Verification items for the finished model (mm, model axes). Face numbers are marked on the shaded views. A direction names the side the tool comes from. Round coordinates to 2 decimals unless told otherwise and drop trailing zeros. Order: outer loops, then holes, each group sorted by start corner. A loop starts at its lowest first (then second) coordinate and runs counter-clockwise, first axis right, second up. Notation, with made-up numbers: M 44,65 L 89,65 A23 cw 89,75 Z; hole C -25.75,69 d11. An arc over 180 degrees is marked long. Use one line per item in the form item = value. Start each with the question number.
Item 1: Thickness scan on probe 1 along X at (y, z) = (-225, 49.5); probe 2 along Y at (x, z) = (25.5, 59); probe 3 along Z at (x, y) = (41, -56.5). Record the ranges inside material, lowest first. Write a range as [from, to].
Item 2: Go/stop test with flat-tipped pins: pin 1 Ø15 at (x, z) = (17, 46) entering from -Y; pin 2 Ø6 at (x, y) = (-54.5, -233) entering from -Z; pin 3 Ø25 at (x, z) = (28, 57.5) entering from +Y. Record where each tip stops, or that it passes through.
Item 3: Release check for a two-part mould opening along Y. For the marked faces 1, 2 and 3 record: +Y half, -Y half, draft (parallel to the pull), parting line (faces both ways), or undercut.
Item 4: Cross-section at D-D on y = -314. Enter the section's corners in (x, z), then the cut area to 3 significant figures.
Item 5: Tool access check on the marked faces 4, 5 and 6. Record the directions out of +Z, -Z, +X, -X, +Y, -Y that give a thin tool (end or side, any length) a straight path to the whole face; none if there is none.
Item 6: Cross-section at B-B on x = -210. Enter the section's corners in (y, z).
Item 7: Cross-section at C-C on y = -175. Enter the section's corners in (x, z).
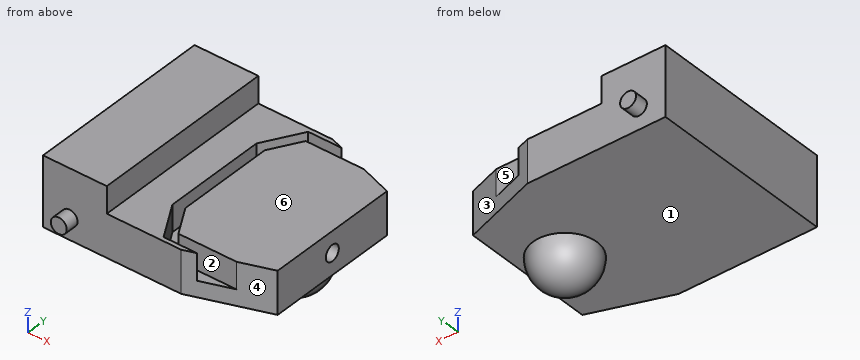
from build123d import *

# Parameters (mm, degrees)
BOSS_EXTRUDE1_DEPTH = 80
SKETCH2_R           = 15
BOSS_EXTRUDE2_DEPTH = 25
BOSS_EXTRUDE3_START = -375
SKETCH2_2_R         = 15
BOSS_EXTRUDE3_DEPTH = 25
SKETCH4_R           = 15
CUT_EXTRUDE1_DEPTH  = 30
CUT_EXTRUDE3_DEPTH  = 50
REVOLVE1_ANGLE      = 180
SKETCH6_W           = 120
SKETCH6_H           = 350
BOSS_EXTRUDE4_DEPTH = 50


with BuildPart() as part:
    # Sketch1 → Boss-Extrude1 (new body)
    with BuildSketch(Plane.XY):
        Polygon((0, 0), (-260, 0), (-260, -350), (0, -350), (141.863078537, -301.267393379), (141.863078537, -48.732606621), align=None)
    extrude(amount=BOSS_EXTRUDE1_DEPTH)

    # Sketch2 → Boss-Extrude2 (add)
    with BuildSketch(Plane.XZ.offset(350)):
        with Locations(Location((-210, 40, 0), (0, 0, 90))):
            Circle(SKETCH2_R)
    extrude(amount=BOSS_EXTRUDE2_DEPTH)

    # Sketch2<2> → Boss-Extrude3 (add)
    with BuildSketch(Plane.XZ.offset(350).offset(BOSS_EXTRUDE3_START)):
        with Locations(Location((-210, 40, 0), (0, 0, 90))):
            Circle(SKETCH2_2_R)
    extrude(amount=BOSS_EXTRUDE3_DEPTH)

    # Sketch4 → Cut-Extrude1 (cut)
    with BuildSketch(Plane(origin=(141.863078537, 0, 0), x_dir=(0, 0, -1), z_dir=(1, 0, 0))):
        with Locations((-40, -175)):
            Circle(SKETCH4_R)
    extrude(amount=-CUT_EXTRUDE1_DEPTH, mode=Mode.SUBTRACT)

    # Sketch5 → Cut-Extrude3 (cut)
    with BuildSketch(Plane.XY.offset(80)):
        Polygon((23.288403945, -342), (-39.585481157, -342), (-80, -272), (-80, -78), (-39.585481157, -8), (23.288403945, -8), (81.509413808, -28), (-28.038475773, -28), (-60, -83.358983849), (-60, -266.641016151), (-28.038475773, -322), (81.509413808, -322), align=None)
    extrude(amount=-CUT_EXTRUDE3_DEPTH, mode=Mode.SUBTRACT)

    # Sketch3 → Revolve1 (revolve)
    with BuildSketch(Plane(origin=(0, 0, 0), x_dir=(-1, 0, 0), z_dir=(0, 0, -1))):
        with BuildLine():
            Line((-11.863078537, -175), (-131.863078537, -175))
            ThreePointArc((-131.863078537, -175), (-71.863078537, -115), (-11.863078537, -175))
        make_face()
    revolve(axis=Axis((141.863078537, -175, 0), (-1, 0, 0)), revolution_arc=REVOLVE1_ANGLE)

    # Sketch6 → Boss-Extrude4 (add)
    with BuildSketch(Plane.XY.offset(80)):
        with Locations((-200, -175)):
            Rectangle(SKETCH6_W, SKETCH6_H)
    extrude(amount=BOSS_EXTRUDE4_DEPTH)


solid = part.part
Output values:
q1.probe_1 = [-260, -80], [-60, 141.86]
q1.probe_2 = [-322, -28]
q1.probe_3 = [0, 80]
q2.pin_1 = -346.74
q2.pin_2 = 0
q2.pin_3 = -5.32
q3.face_1 = draft
q3.face_2 = undercut
q3.face_3 = +Y half
q4.outline = M -260,0 L 104.8,0 L 104.8,80 L -32.66,80 L -32.66,30 L -55.75,30 L -55.75,80 L -140,80 L -140,130 L -260,130 Z
q4.area = 34,000 mm2
q5.face_4 = +Z, -Z, +X, -Y
q5.face_5 = +Z, +X
q5.face_6 = +Z, +X, +Y, -Y
q6.outline = M -375,25 L -350,25 L -350,0 L 0,0 L 0,25 L 25,25 L 25,55 L 0,55 L 0,130 L -350,130 L -350,55 L -375,55 Z
q7.outline = M -260,0 L 11.86,0 A60 ccw 131.86,0 L 141.86,0 L 141.86,25 L 111.86,25 L 111.86,55 L 141.86,55 L 141.86,80 L -60,80 L -60,30 L -80,30 L -80,80 L -140,80 L -140,130 L -260,130 Z
